Input: part model. Units: mm. Frame: model coordinates. A direction names the side the tool comes from. Give positions to 0.01 mm unless a question says otherwise; leave off trailing zeros. Loops run counter-clockwise (first coordinate to the right, second up) from the corner with the lowest first, then second, coordinate; pieces in that order, holes last. Notation, with made-up numbers: (-38, -19.5) - (-31, -19.5) arc R26 ccw to (-31, 8.5) - close; hole circle Ø7 at (16, 22.5). An arc over 180 degrees is marked (long way). Answer as a JSON object with one key per item and string values.
from build123d import *

# Parameters (mm, degrees)
BOSS_EXTRUDE1_DEPTH = 6
CHAMFER1_DEPTH      = 6
CUT_EXTRUDE1_DEPTH  = 6


with BuildPart() as part:
    # Sketch1 → Boss-Extrude1 (new body)
    with BuildSketch(Plane.XY):
        with BuildLine():
            Line((5, -3), (5, 0))
            Line((5, 0), (7.999917137, -0.022297349))
            Line((7.999917137, -0.022297349), (24.574810766, 33.988914515))
            ThreePointArc((24.574810766, 33.988914515), (24.906699983, 38.765486885), (21.826463092, 42.431265759))
            add(Edge.make_bspline(
                [(21.826463092, 42.431265759), (4.303477857, 50.343378655), (-29.026405502, 57.018304793), (-62.241820335, 50.620507444), (-77.999999998, 43.5)],
                knots=[0.018384898, 0.018384898, 0.018384898, 0.018384898, 0.528855814, 0.991084545, 0.991084545, 0.991084545, 0.991084545], degree=3))
            Line((-77.999999998, 43.5), (-77.999999998, 40.5))
            Line((-77.999999998, 40.5), (-81, 40.5))
            Line((-81, 40.5), (-81, 35.5))
            Line((-81, 35.5), (-78, 35.5))
            add(Edge.make_bspline(
                [(17.092660216, 35.073654222), (-30.383266578, 55.711591107), (-78, 35.5)],
                knots=[0, 0, 0, 1, 1, 1], degree=2))
            Line((17.092660216, 35.073654222), (0, 0))
            Line((0, 0), (0, -3))
            Line((0, -3), (5, -3))
        make_face()
    extrude(amount=BOSS_EXTRUDE1_DEPTH)

    # Chamfer1: read off the stored shape, not the designer's step
    # Chamfer1 outline → Chamfer1 (add)
    with BuildSketch(Plane.XY):
        with BuildLine():
            Line((8.096256687, 38.617267247), (12.890218446, 26.45036284))
            Line((12.890218446, 26.45036284), (17.092660216, 35.073654222))
            add(Edge.make_bspline(
                [(17.092660216, 35.073654222), (12.595090284, 37.028762224), (8.096256687, 38.617267247)],
                knots=[0, 0, 0, 0.094733694, 0.094733694, 0.094733694], degree=2))
        make_face()
    extrude(amount=CHAMFER1_DEPTH)

    # Sketch4 → Cut-Extrude1 (cut)
    with BuildSketch(Plane.XY.offset(6)):
        Polygon((8.369117538, 12.607849604), (12.74995002, 21.597193671), (15.44675324, 20.282943927), (11.065920758, 11.293599859), align=None)
    extrude(amount=-CUT_EXTRUDE1_DEPTH, mode=Mode.SUBTRACT)


solid = part.part
Item 1: Access query for faces 1 (the face through (-80, 35.5, 3)), 2 (the face through (-78, 42, 3)), 3 (the face through (10.46, 32.62, 2.96)), 4 (the face through (5, -2, 3)). Directions: +Z, -Z, +X, -X, +Y, -Y. A direction counts if a zero-diameter tool reaches every point of the face in a straight line with its end or side. Return the directions, or none.
Geometry check:
{"face 1": "+Z, -Z, -X, -Y", "face 2": "+Z, -Z, -X, +Y", "face 3": "+Z, -Z", "face 4": "+Z, -Z, +X, -Y"}
Item 2: Mould query, pull axis Y, two halves, no side actions, for faces 5 (the face through (-79, 40.5, 3)), 6 (the face through (6.535, 13.41, 2.958)), 7 (the face through (16.171, 16.745, 2.958)). Classes: released by +Y, released by -Y, zero draft, split by the parting line, or undercut.
Geometry check:
{"face 5": "released by +Y", "face 6": "undercut", "face 7": "released by -Y"}
Item 3: Material intervals for line 1 (X direction, y = 20, z = 2.25); line 2 (X direction, y = 18, z = 2.25); line 3 (Y direction, x = 1, z = 1), sorted ascending. Write a range as [from, to].
Geometry check:
{"line 1": "x = [9.75, 11.97], [15.31, 17.76]", "line 2": "x = [8.77, 11], [14.33, 16.78]", "line 3": "y = [-3, 2.05], [40.89, 49.81]"}
Item 4: Contact query for flat-ended pins moving along their axis: P1, Ø0.9, axis at x = -79, z = 2.5, coming from the +Y side; P2, Ø0.9, axis at y = -2, z = 2.5, coming from the -X side; P3, Ø2, axis at x = -26, z = 2.5, coming from the +Y side. Output: stop coordinate, or through.
Geometry check:
{"P1": "stops at y = 40.5", "P2": "stops at x = 0", "P3": "stops at y = 53.72"}
Item 5: Cut plane A-A (y = 6). Return loops of the section in (x, z).
Geometry check:
{"outline": "(2.92, 0) - (10.93, 0) - (10.93, 6) - (2.92, 6) - close"}
